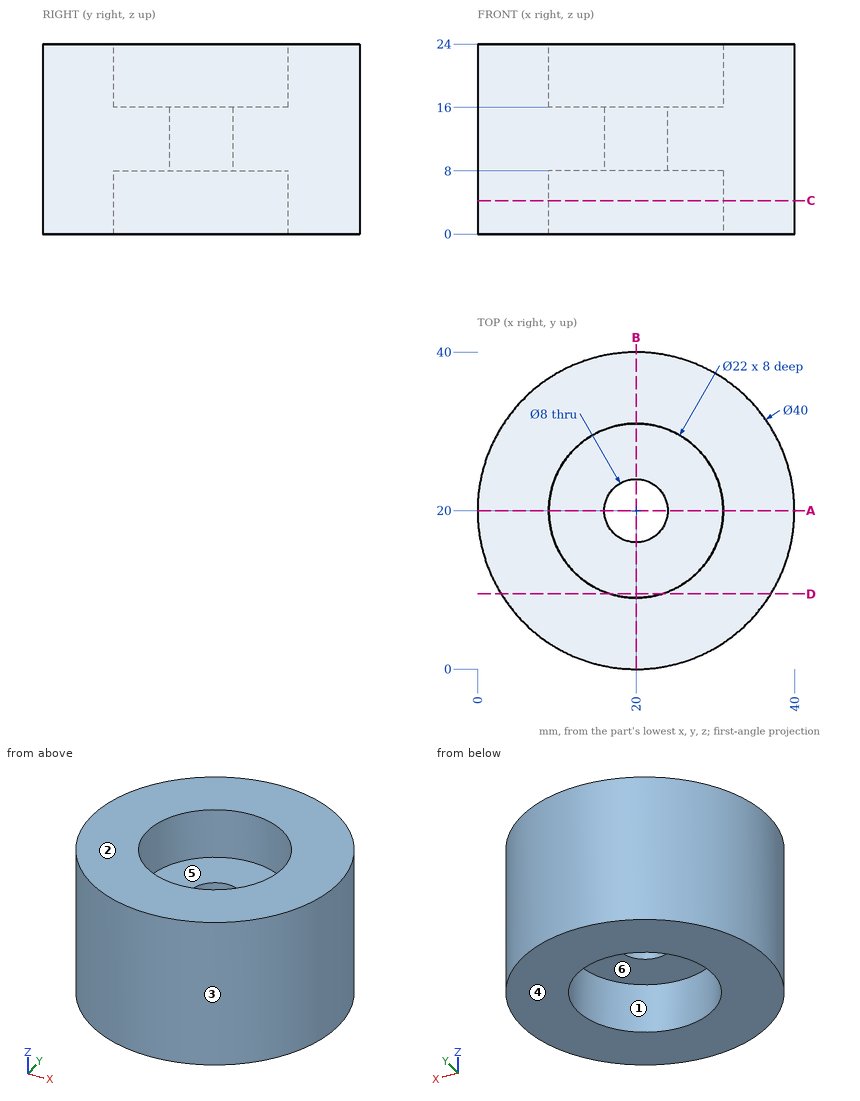
Design review of the part shown in the three views and the two pictorial views. Dimensions are in mm from the part's minimum x, y and z. A direction names the side the tool comes from. Give positions to 0.01 mm unless a question says otherwise; leave off trailing zeros. Write each loop counter-clockwise with the first axis right and the second up, starting at its lowest first coordinate (ties: lowest second). Pieces come first, ordered by that corner, then holes.
Item 1: Wall thickness on probe 1 along Y at (x, z) = (20, 21.75); probe 2 along Z at (x, y) = (15, 29.5); probe 3 along Y at (x, z) = (23.5, 3.25): over which ranges is each line inside the solid? List them lowest first.
Item 2: Take a section at C-C (z = 4.25). Give the boundary of the cut face in (x, y), and give its area (3 significant figures).
Item 3: Take a section at D-D (y = 9.5). Give the boundary of the cut face in (x, z).
Item 4: The part is to be moulded in two halves that separate along Y. For the marked faces 1, 2 and 3, say which applies: +Y half, -Y half, draft (parallel to the pull), parting line (faces both ways), or undercut.
Item 5: Take a section at A-A (y = 20). Give the boundary of the cut face in (x, z).
Item 6: Insertion check: P1, Ø20, axis at x = 20, y = 20, coming from the -Z side; P2, Ø8, axis at x = 7.5, z = 4.5, coming from the +Y side; P3, Ø1, axis at y = 23.5, z = 12, coming from the +X side. Each pin has a flat end and moves straight along its axis. Give the tip position at first contact, or say it passes through.
Item 7: Machinability: for the marked faces 4, 5 and 6, which of the approach directions +Z, -Z, +X, -X, +Y, -Y give a long, thin tool a straight path to every point of the face, cutting with its end or side? Answer none if there is none.
Established:
1. probe 1: y = 0 to 9, 31 to 40
1. probe 2: z = 8 to 16
1. probe 3: y = 0.31 to 9.57, 30.43 to 39.69
2. outline: circle Ø40 at (20, 20); hole circle Ø22 at (20, 20)
2. area: 877 mm2
3. outline: (2.98, 0) - (16.72, 0) - (16.72, 8) - (23.28, 8) - (23.28, 0) - (37.02, 0) - (37.02, 24) - (23.28, 24) - (23.28, 16) - (16.72, 16) - (16.72, 24) - (2.98, 24) - close
4. face 1: undercut
4. face 2: draft
4. face 3: parting line
5. outline: (0, 0) - (9, 0) - (9, 8) - (16, 8) - (16, 16) - (9, 16) - (9, 24) - (0, 24) - close; (24, 8) - (31, 8) - (31, 0) - (40, 0) - (40, 24) - (31, 24) - (31, 16) - (24, 16) - close
6. P1: stops at z = 8
6. P2: stops at y = 38.1
6. P3: stops at x = 39.77
7. face 4: -Z, +X, -X, +Y, -Y
7. face 5: +Z
7. face 6: -Z
